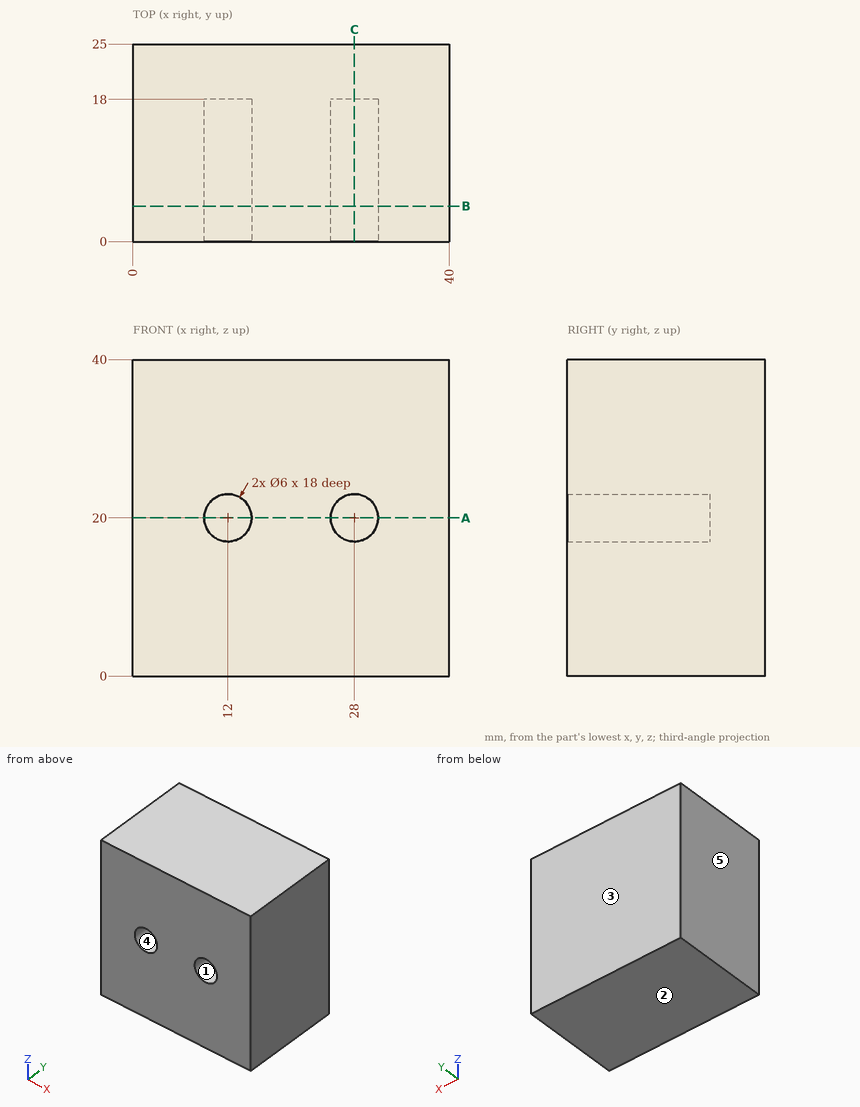
Design review of the part shown in the three views and the two pictorial views. Dimensions are in mm from the part's minimum x, y and z. A direction names the side the tool comes from. Round coordinates to 2 decimals unless told otherwise and drop trailing zeros. Order: outer loops, then holes, each group sorted by start corner. A loop starts at its lowest first (then second) coordinate and runs counter-clockwise, first axis right, second up. Notation, with made-up numbers: M -23.75,-20.75 L -0.75,-20.75 A32 cw -0.75,17.25 Z; hole C 85,77 d6. An arc over 180 degrees is marked long. Put each result on its own line as item: value.
Q1. To check wall thickness, follow line 1 (X direction, y = 14, z = 20); line 2 (X direction, y = 14.25, z = 22.5); line 3 (Z direction, x = 9.5, y = 10). State the ranges of each line that lie inside material, in increasing order.
Reported:
line 1: 0 to 9, 15 to 25, 31 to 40
line 2: 0 to 10.34, 13.66 to 26.34, 29.66 to 40
line 3: 0 to 18.34, 21.66 to 40
Q2. Consider section B-B (y = 4.5). State the section outline as (x, z) points, and give its area (3 significant figures).
Reported:
outline: M 0,0 L 40,0 L 40,40 L 0,40 Z; hole C 12,20 d6; hole C 28,20 d6
area: 1,540 mm²
Q3. Consider section A-A (z = 20). State the section outline as (x, y) points.
Reported:
outline: M 0,0 L 9,0 L 9,18 L 15,18 L 15,0 L 25,0 L 25,18 L 31,18 L 31,0 L 40,0 L 40,25 L 0,25 Z
Q4. Insertion check: pin 1 Ø3.5 at (x, z) = (28, 20) entering from -Y. The pin has a flat end and moves straight along its axis. Give the tip position at first contact, or say it passes through.
Reported:
pin 1: y = 18
Q5. Draft analysis for pull direction X (two halves, no side actions). For the marked faces 3, 4 and 5, state which applies: released by +X, released by -X, zero draft, split by the parting line, or undercut.
Reported:
face 3: zero draft
face 4: undercut
face 5: released by -X
Q6. Machinability: for the marked faces 1 and 2, which of the approach directions +Z, -Z, +X, -X, +Y, -Y give a long, thin tool a straight path to every point of the face, cutting with its end or side? Answer none if there is none.
Reported:
face 1: -Y
face 2: -Z, +X, -X, +Y, -Y
Q7. Consider section C-C (x = 28). State the section outline as (y, z) points.
Reported:
outline: M 0,0 L 25,0 L 25,40 L 0,40 L 0,23 L 18,23 L 18,17 L 0,17 Z
